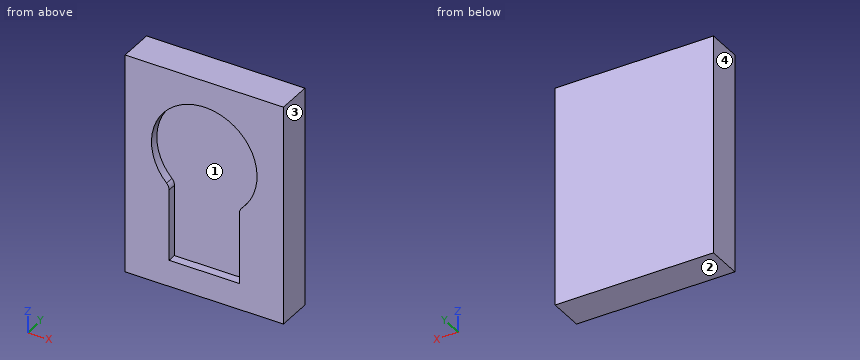
from build123d import *

# Parameters (mm, degrees)
SKETCH1_W           = 18
SKETCH1_H           = 25
BOSS_EXTRUDE1_DEPTH = 1
SKETCH2_W           = 18
SKETCH2_H           = 25
BOSS_EXTRUDE2_DEPTH = 3


with BuildPart() as part:
    # Sketch1 → Boss-Extrude1 (new body)
    with BuildSketch(Plane(origin=(0, 0, 0), x_dir=(1, 0, 0), z_dir=(0, 1, 0))):
        with Locations((0, 3.5)):
            Rectangle(SKETCH1_W, SKETCH1_H)
        with BuildLine():
            Line((-4, 13), (4, 13))
            Line((4, 13), (4, 5.5))
            Line((4, 5.5), (4, 4.898979486))
            ThreePointArc((4, 4.898979486), (4.0741799, 4.521015013), (4.285714286, 4.199125273))
            ThreePointArc((4.285714286, 4.199125273), (0, -6), (-4.285714286, 4.199125273))
            ThreePointArc((-4.285714286, 4.199125273), (-4.0741799, 4.521015013), (-4, 4.898979486))
            Line((-4, 4.898979486), (-4, 5.5))
            Line((-4, 5.5), (-4, 13))
        make_face(mode=Mode.SUBTRACT)
    extrude(amount=BOSS_EXTRUDE1_DEPTH)

    # Sketch2 → Boss-Extrude2 (add)
    with BuildSketch(Plane(origin=(0, 1, 0), x_dir=(1, 0, 0), z_dir=(0, 1, 0))):
        with Locations((0, 3.5)):
            Rectangle(SKETCH2_W, SKETCH2_H)
    extrude(amount=BOSS_EXTRUDE2_DEPTH)


solid = part.part
Can you work these out from the model? Positions are in its coordinate system, mm. Face numbers are marked on the shaded views. Round coordinates to 2 decimals unless told otherwise and drop trailing zeros. Loops run counter-clockwise (first coordinate to the right, second up) from the corner with the lowest first, then second, coordinate; pieces in that order, holes last. Notation, with made-up numbers: (5.5, -11) - (56.5, -11) arc R28 ccw to (56.5, 10) - close; hole circle Ø9 at (47.25, -8). An arc over 180 degrees is marked (long way). Answer in a Markdown table with one row per item. Add a question column.
Q1. I need wall thicknesses on L1, parallel to Z at x = 0, y = 0.7; L2, parallel to X at y = 0.3, z = 0; L3, parallel to Y at x = 1.25, z = 5.75. Which ranges of each line are inside material? Lowest first, please.
Q2. For pin 1 Ø3.5 at (x, z) = (1, -3.5) entering from -Y, with a flat end and sliding along its axis, tell me the tip position at first contact or that it passes through.
Q3. I want a section at B-B on z = -6.25. List the corners of the cut face in (x, y) for me.
Q4. We'd pull the mould along X, two halves only. Please class the marked faces 1, 2, 3 and 4: pulls with the +X half, pulls with the -X half, needs draft (parallel to the pull), parting line crosses it, or undercut.
Q5. I want a section at C-C on x = 0. List the corners of the cut face in (y, z) for me, and give its area (3 significant figures).
Q6. I want a section at A-A on y = 0.3. List the corners of the cut face in (x, z) for me, and give its area (3 significant figures).
A:
| question | item | result |
|---|---|---|
| 1 | L1 | -16 to -13, 6 to 9 |
| 1 | L2 | -9 to -6, 6 to 9 |
| 1 | L3 | 1 to 4 |
| 2 | pin 1 | y = 1 |
| 3 | outline | (-9, 0) - (-4, 0) - (-4, 1) - (4, 1) - (4, 0) - (9, 0) - (9, 4) - (-9, 4) - close |
| 4 | face 1 | undercut |
| 4 | face 2 | needs draft |
| 4 | face 3 | pulls with the +X half |
| 4 | face 4 | pulls with the -X half |
| 5 | outline | (0, -16) - (4, -16) - (4, 9) - (0, 9) - (0, 6) - (1, 6) - (1, -13) - (0, -13) - close |
| 5 | area | 81.0 mm^2 |
| 6 | outline | (-9, -16) - (9, -16) - (9, 9) - (-9, 9) - close; hole (-4.29, -4.2) arc R1 cw to (-4, -4.9) - (-4, -13) - (4, -13) - (4, -4.9) arc R1 cw to (4.29, -4.2) arc R6 ccw (long way) to start |
| 6 | area | 277 mm^2 |
